from build123d import *

# Parameters (mm, degrees)
SKETCH2_R           = 5
SKETCH2_W           = 3
SKETCH2_H           = 3
BOSS_EXTRUDE2_DEPTH = 3


with BuildPart() as part:
    # Sketch2 → Boss-Extrude2 (new body)
    with BuildSketch(Plane.XY):
        Circle(SKETCH2_R)
        Rectangle(SKETCH2_W, SKETCH2_H, mode=Mode.SUBTRACT)
    extrude(amount=BOSS_EXTRUDE2_DEPTH)


solid = part.part
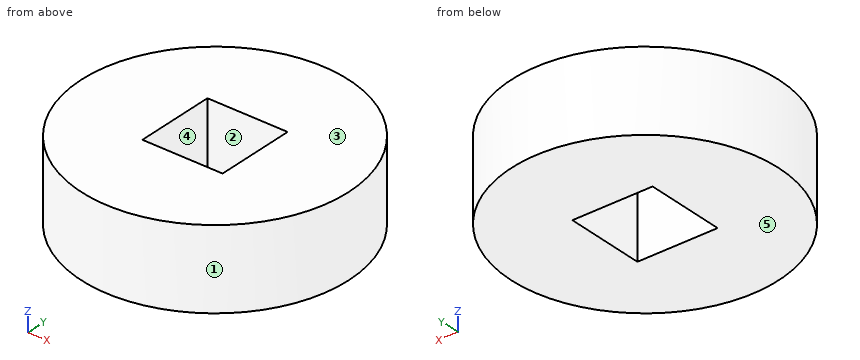
Design review of the part built by this model. Coordinates are the model's own, in mm. Face numbers are marked on the shaded views. A direction names the side the tool comes from. Coordinates: 2 decimals unless noted, no trailing zeros. Loops run counter-clockwise (first coordinate to the right, second up) from the corner with the lowest first, then second, coordinate; pieces in that order, holes last.
Item 1: Add section D-D (y = 4). Write out the cut boundary in (x, z), and give its area (3 significant figures).
Completed:
outline: (-3, 0) - (3, 0) - (3, 3) - (-3, 3) - close
area: 18.0 mm2
Item 2: Add section A-A (y = 0). Write out the cut boundary in (x, z), and give its area (3 significant figures).
Completed:
outline: (-5, 0) - (-1.5, 0) - (-1.5, 3) - (-5, 3) - close; (1.5, 0) - (5, 0) - (5, 3) - (1.5, 3) - close
area: 21.0 mm2
Item 3: Add section C-C (z = 2.5). Write out the cut boundary in (x, y).
Completed:
outline: circle Ø10 at (0, 0); hole (-1.5, -1.5) - (1.5, -1.5) - (1.5, 1.5) - (-1.5, 1.5) - close
Item 4: For the marked faces 4 and 5, list the 3-axis set-ups (+Z, -Z, +X, -X, +Y, -Y) from which the entire face can be reached by the end or side of a thin tool; tool diameter is ignored.
Completed:
face 4: +Z, -Z
face 5: -Z, +X, -X, +Y, -Y
Item 5: Wall thickness on L1, parallel to X at y = 1, z = 2.9; L2, parallel to Y at x = -0.5, z = 1.75; L3, parallel to X at y = 1.25, z = 1.2: over which ranges is each line inside the solid? List them lowest first.
Completed:
L1: x = -4.9 to -1.5, 1.5 to 4.9
L2: y = -4.97 to -1.5, 1.5 to 4.97
L3: x = -4.84 to -1.5, 1.5 to 4.84
Item 6: Draft analysis for pull direction X (two halves, no side actions). For the marked faces 1, 2 and 3, state which applies: pulls with the +X half, pulls with the -X half, needs draft (parallel to the pull), parting line crosses it, or undercut.
Completed:
face 1: parting line crosses it
face 2: undercut
face 3: needs draft
